Geometry: final body of the model. Coordinates: model frame, mm. A direction names the side the tool comes from. Give positions to 0.01 mm unless a question says otherwise; leave off trailing zeros. Loops run counter-clockwise (first coordinate to the right, second up) from the corner with the lowest first, then second, coordinate; pieces in that order, holes last. Notation, with made-up numbers: (-13, 73) - (3, 73) arc R22 cw to (3, 79) - close; hole circle Ø7 at (-21, 2). An arc over 180 degrees is marked (long way). Answer in a Markdown table with one row per item.
from build123d import *

# Parameters (mm, degrees)
ESQUISSE1_W             = 600
ESQUISSE1_H             = 150
BOSS_EXTRU_1_DEPTH      = 18
ESQUISSE3_W             = 42
ESQUISSE3_H             = 42
ENL_V_MAT_EXTRU_1_DEPTH = 20


with BuildPart() as part:
    # Esquisse1 → Boss.-Extru.1 (new body)
    with BuildSketch(Plane(origin=(0, 0, 0), x_dir=(1, 0, 0), z_dir=(0, 1, 0))):
        Rectangle(ESQUISSE1_W, ESQUISSE1_H)
    extrude(amount=BOSS_EXTRU_1_DEPTH)

    # Esquisse3 → Enlèv. mat.-Extru.1 (cut)
    with BuildSketch(Plane(origin=(0, 18, 0), x_dir=(1, 0, 0), z_dir=(0, 1, 0))):
        with Locations((-269, -54)):
            Rectangle(ESQUISSE3_W, ESQUISSE3_H)
        with Locations((269, -54)):
            Rectangle(ESQUISSE3_W, ESQUISSE3_H)
    extrude(amount=-ENL_V_MAT_EXTRU_1_DEPTH, mode=Mode.SUBTRACT)


solid = part.part
Q1. First-contact query: pin 1 (9 mm diameter, centred on x = -263, y = 10, fed in from +Z); pin 2 (2 mm diameter, centred on x = -123, z = -48, fed in from -Y). Flat tips, straight axial feed; report the tip coordinate or a pass-through.
Check values:
| item | result |
|---|---|
| pin 1 | z = 33 |
| pin 2 | y = 0 |
Q2. Draft query along X for faces 1 (the flat face through (-300, 9, 1)), 2 (the flat face through (-295, 9, 75)), 3 (the flat face through (269, 9, 33)). Return one class per face: pulls with the +X half, pulls with the -X half, needs draft (parallel to the pull), parting line crosses it, or undercut.
Check values:
| item | result |
|---|---|
| face 1 | pulls with the -X half |
| face 2 | needs draft |
| face 3 | undercut |
Q3. Cut plane A-A (z = 58.5). Output: boundary loops of the cut face in (x, y).
Check values:
| item | result |
|---|---|
| outline | (-300, 0) - (-290, 0) - (-290, 18) - (-300, 18) - close; (-248, 0) - (248, 0) - (248, 18) - (-248, 18) - close; (290, 0) - (300, 0) - (300, 18) - (290, 18) - close |
Q4. Reachability of faces 4 (the flat face through (295, 9, 75)), 5 (the flat face through (-290, 9, 54)) from +Z, -Z, +X, -X, +Y, -Y: full face, straight path, thin tool, end or side. Return the list, or none.
Check values:
| item | result |
|---|---|
| face 4 | +Z, +X, -X, +Y, -Y |
| face 5 | +Z, +Y, -Y |
Q5. Cut plane B-B (y = 4.75). Output: boundary loops of the cut face in (x, z), and give its area (3 significant figures).
Check values:
| item | result |
|---|---|
| outline | (-300, -75) - (300, -75) - (300, 75) - (290, 75) - (290, 33) - (248, 33) - (248, 75) - (-248, 75) - (-248, 33) - (-290, 33) - (-290, 75) - (-300, 75) - close |
| area | 86,500 mm² |
Q6. Material intervals for line 1 along X through (y, z) = (15.5, 44); line 2 along Z through (x, y) = (260.5, 16), sorted ascending.
Check values:
| item | result |
|---|---|
| line 1 | -300 to -290, -248 to 248, 290 to 300 |
| line 2 | -75 to 33 |
